from build123d import *

# Parameters (mm, degrees)
SKETCH1_R           = 1.651
BOSS_EXTRUDE1_DEPTH = 3.048
FILLET3_R           = 4
CHAMFER1_SIZE       = 1.3
FILLET4_R           = 6


with BuildPart() as part:
    # Sketch1 → Boss-Extrude1 (new body)
    with BuildSketch(Plane(origin=(0, 0, 0), x_dir=(1, 0, 0), z_dir=(0, 1, 0))):
        Polygon((-24.895, 4.064), (-4.064, 4.064), (-4.064, 24.895), (4.064, 24.895), (4.064, 4.064), (24.895, 4.064), (24.895, -4.064), (4.064, -4.064), (4.064, -24.895), (-4.064, -24.895), (-4.064, -4.064), (-24.895, -4.064), align=None)
        with Locations((21.025, 0)):
            Circle(SKETCH1_R, mode=Mode.SUBTRACT)
        with Locations((0, 21.025)):
            Circle(SKETCH1_R, mode=Mode.SUBTRACT)
        with Locations((-21.025, 0)):
            Circle(SKETCH1_R, mode=Mode.SUBTRACT)
        with Locations((0, -21.025)):
            Circle(SKETCH1_R, mode=Mode.SUBTRACT)
    extrude(amount=BOSS_EXTRUDE1_DEPTH)

    # Fillet3
    fillet3_edges = [part.edges().sort_by_distance(p)[0] for p in [
        (4.064, 1.524, 24.895),
        (-4.064, 1.524, 24.895),
        (-24.895, 1.524, 4.064),
        (-24.895, 1.524, -4.064),
        (-4.064, 1.524, -24.895),
        (4.064, 1.524, -24.895),
        (24.895, 1.524, -4.064),
        (24.895, 1.524, 4.064),
    ]]
    fillet(fillet3_edges, radius=FILLET3_R)

    # Chamfer1
    chamfer1_edges = [part.edges().sort_by_distance(p)[0] for p in [
        (19.374, 3.048, 0),
        (-1.651, 3.048, -21.025),
        (-22.676, 3.048, 0),
        (-1.651, 3.048, 21.025),
    ]]
    chamfer(chamfer1_edges, length=CHAMFER1_SIZE)

    # Fillet4
    fillet4_edges = [part.edges().sort_by_distance(p)[0] for p in [
        (4.064, 1.524, 4.064),
        (-4.064, 1.524, 4.064),
        (-4.064, 1.524, -4.064),
        (4.064, 1.524, -4.064),
    ]]
    fillet(fillet4_edges, radius=FILLET4_R)


solid = part.part
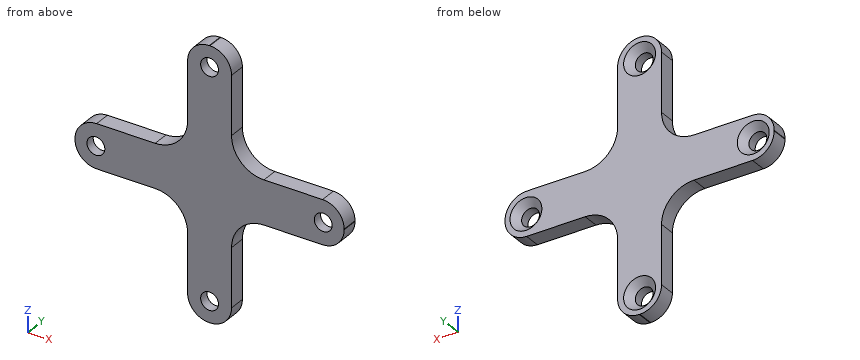
Can you work these out from the model? Positions are in its coordinate system, mm. Coordinates: 2 decimals unless noted, no trailing zeros. Loops run counter-clockwise (first coordinate to the right, second up) from the corner with the lowest first, then second, coordinate; pieces in that order, holes last. Notation, with made-up numbers: M 55.5,80.5 L 105.5,80.5 A22 ccw 105.5,99.5 Z; hole C 0.5,-6 d1. An arc over 180 degrees is marked long. Return JSON: item names as keys, results as strings. Group by question number.
Item 1: Imagine slicing it at C-C (x = 12.5). Please give me the cut outline in (y, z), and give its area (3 significant figures).
Item 2: Imagine slicing it at A-A (y = 1.1). Please give me the cut outline in (x, z) (3 decimals).
Item 3: I'm going to push flat-ended pins straight in: pin 1 Ø1 at (x, y) = (11.5, 2) entering from +Z; pin 2 Ø0.9 at (y, z) = (1, 17.5) entering from +X; pin 3 Ø4 at (x, z) = (0, 21.025) entering from +Y. Where does each tip first touch, or does it pass through?
Item 4: Imagine slicing it at B-B (z = -15). Please give me the cut outline in (x, y), and give its area (3 significant figures).
Item 5: If I drill on L1, parallel to Z at x = 0, y = 1.35 (3 decimals); L2, parallel to X at y = 1.8, z = 15, over which ranges is the centre line in solid material (lowest first)? Write a range as from..to.
Verdict:
{
 "1": {"outline": "M 0,-4.06 L 3.05,-4.06 L 3.05,4.06 L 0,4.06 Z", "area": "24.8 mm^2"},
 "2": {"outline": "M -24.895,-0.064 A4 ccw -20.895,-4.064 L -10.064,-4.064 A6 cw -4.064,-10.064 L -4.064,-20.895 A4 ccw -0.064,-24.895 L 0.064,-24.895 A4 ccw 4.064,-20.895 L 4.064,-10.064 A6 cw 10.064,-4.064 L 20.895,-4.064 A4 ccw 24.895,-0.064 L 24.895,0.064 A4 ccw 20.895,4.064 L 10.064,4.064 A6 cw 4.064,10.064 L 4.064,20.895 A4 ccw 0.064,24.895 L -0.064,24.895 A4 ccw -4.064,20.895 L -4.064,10.064 A6 cw -10.064,4.064 L -20.895,4.064 A4 ccw -24.895,0.064 Z; hole C -21.025,0 d3.302; hole C 0,-21.025 d3.302; hole C 0,21.025 d3.302; hole C 21.025,0 d3.302"},
 "3": {"pin 1": "stops at z = 4.06", "pin 2": "stops at x = 4.06", "pin 3": "stops at y = 2.1"},
 "4": {"outline": "M -4.06,0 L 4.06,0 L 4.06,3.05 L -4.06,3.05 Z", "area": "24.8 mm^2"},
 "5": {"L1": "z = -24.895..-22.676, -19.374..19.374, 22.676..24.895", "L2": "x = -4.06..4.06"}
}
